Check sheet for the drawn part. Datum: minimum x, y, z corner. Units: mm. Give positions to 0.01 mm unless a question says otherwise; leave off trailing zeros. Order: outer loops, then holes, each group sorted by start corner. A loop starts at its lowest first (then second) coordinate and runs counter-clockwise, first axis right, second up.
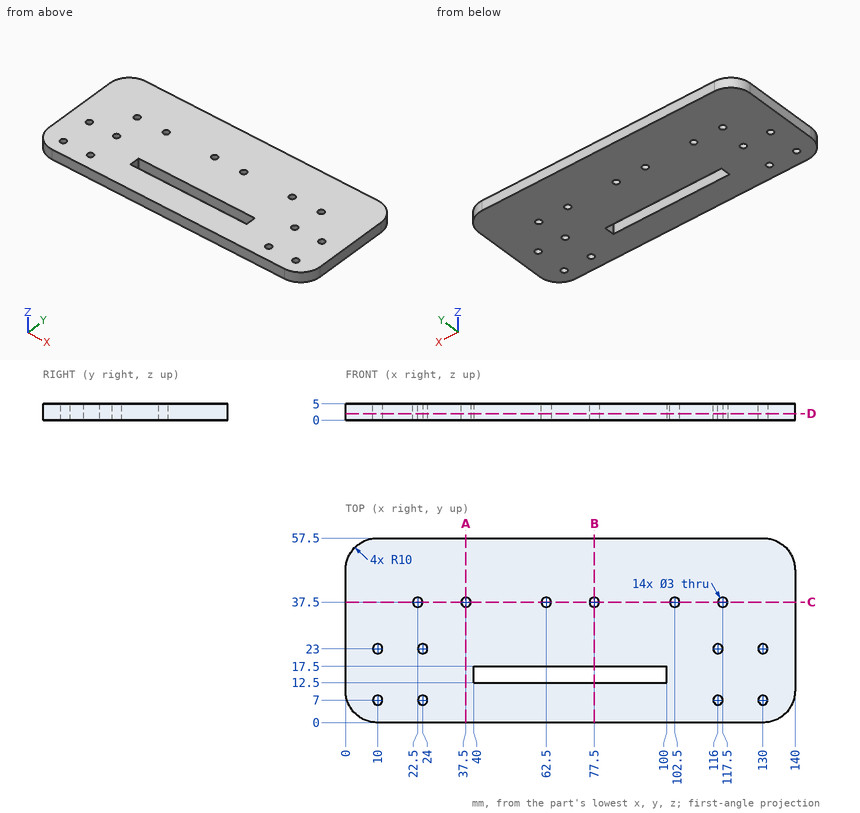
Item 1: Gauge pin test, flat end, axial feed: pin 1 (3 mm diameter, centred on y = 51, z = 3.5, fed in from +X). Record the tip position at first contact, or that the pin passes through.
Reported:
pin 1: stops at x = 139.8
Item 2: Scan lines: L1, parallel to Y at x = 130, z = 2.9; L2, parallel to Y at x = 77.5, z = 3.05; L3, parallel to Y at x = 74.5, z = 3.2. Record each from-to range of solid material in increasing order.
Reported:
L1: y = 0 to 5.5, 8.5 to 21.5, 24.5 to 57.5
L2: y = 0 to 12.5, 17.5 to 36, 39 to 57.5
L3: y = 0 to 12.5, 17.5 to 57.5
Item 3: Sectioned sample at C-C (y = 37.5). Enter the section's corners in (x, z), and give its area (3 significant figures).
Reported:
outline: (0, 0) - (21, 0) - (21, 5) - (0, 5) - close; (24, 0) - (36, 0) - (36, 5) - (24, 5) - close; (39, 0) - (61, 0) - (61, 5) - (39, 5) - close; (64, 0) - (76, 0) - (76, 5) - (64, 5) - close; (79, 0) - (101, 0) - (101, 5) - (79, 5) - close; (104, 0) - (116, 0) - (116, 5) - (104, 5) - close; (119, 0) - (140, 0) - (140, 5) - (119, 5) - close
area: 610 mm2
Item 4: Sectioned sample at A-A (x = 37.5). Enter the section's corners in (y, z).
Reported:
outline: (0, 0) - (36, 0) - (36, 5) - (0, 5) - close; (39, 0) - (57.5, 0) - (57.5, 5) - (39, 5) - close
Item 5: Sectioned sample at B-B (x = 77.5). Enter the section's corners in (y, z).
Reported:
outline: (0, 0) - (12.5, 0) - (12.5, 5) - (0, 5) - close; (17.5, 0) - (36, 0) - (36, 5) - (17.5, 5) - close; (39, 0) - (57.5, 0) - (57.5, 5) - (39, 5) - close
Item 6: Sectioned sample at D-D (z = 2). Give the number of separate pieces and of enclosed holes in the cut face, and give its area (3 significant figures).
Reported:
separate pieces: 1
enclosed holes: 15
area: 7,570 mm2
